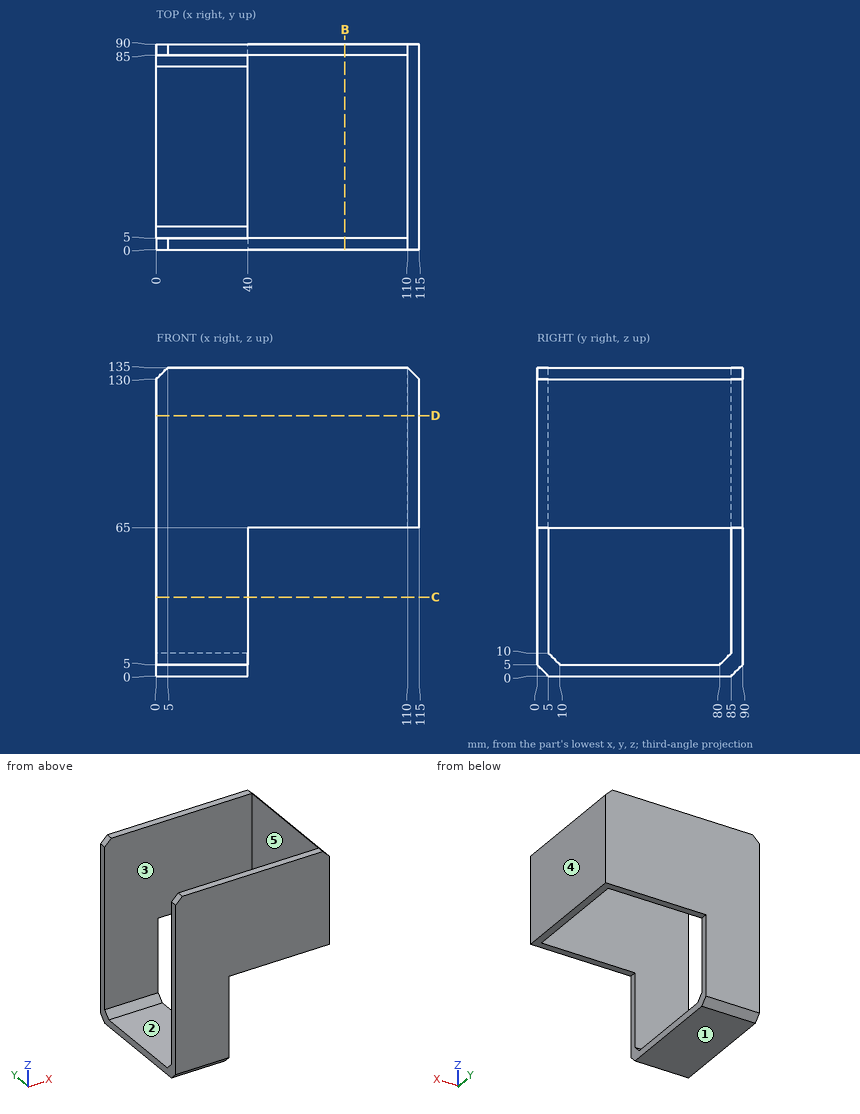
Print and shaded views of the part. All mm, measured from the part's lowest x, y and z. A direction names the side the tool comes from. Round coordinates to 2 decimals unless told otherwise and drop trailing zeros. Write each loop counter-clockwise with the first axis right and the second up, starting at its lowest first coordinate (ties: lowest second). Pieces come first, ordered by that corner, then holes. Notation, with made-up numbers: (-16, -36.75) - (24, -36.75) arc R38 ccw to (24, 2.25) - close; hole circle Ø7 at (-31.5, 83.5). An arc over 180 degrees is marked (long way). One line per item, written item: value.
(1) Cut at D-D, the plane z = 114. Give the cut face in (x, y).
Values follow:
outline: (0, 0) - (115, 0) - (115, 90) - (0, 90) - (0, 85) - (110, 85) - (110, 5) - (0, 5) - close
(2) Cut at C-C, the plane z = 34.5. Give the cut face in (x, y).
Values follow:
outline: (0, 0) - (40, 0) - (40, 5) - (0, 5) - close; (0, 85) - (40, 85) - (40, 90) - (0, 90) - close
(3) Cut at B-B, the plane x = 82.5. Give the cut face in (y, z).
Values follow:
outline: (0, 65) - (5, 65) - (5, 135) - (0, 135) - close; (85, 65) - (90, 65) - (90, 135) - (85, 135) - close
(4) Wall check: probe 1 along Y at (x, z) = (105, 89); probe 2 along X at (y, z) = (52, 85); probe 3 along X at (y, z) = (4, 28.5). Give the ranges that are in metal, low to high.
Values follow:
probe 1: y = 0 to 5, 85 to 90
probe 2: x = 110 to 115
probe 3: x = 0 to 40
(5) 3-axis set-ups, long thin cutter, end or side, ignore diameter. For the marked faces 1, 2, 3, 4 and 5: which of +Z, -Z, +X, -X, +Y, -Y reach the whole face in a straight line?
Values follow:
face 1: -Z, +X, -X, +Y, -Y
face 2: +Z, +X, -X
face 3: +Z, -X
face 4: +Z, -Z, +X, +Y, -Y
face 5: +Z, -Z, -X
(6) Drop flat-ended pins along their axis: P1, Ø5, axis at y = 18, z = 103, coming from the -X side; P2, Ø12, axis at x = 14, y = 54.5, coming from the +Z side; P3, Ø22.5, axis at x = 60.5, y = 27, coming from the -Z side. Give the stop position or say it passes through.
Values follow:
P1: stops at x = 110
P2: stops at z = 5
P3: passes through
